Could you check a few things on this model? Use its own coordinates, in mm. Face numbers are marked on the shaded views. Round coordinates to 2 decimals unless told otherwise and drop trailing zeros. Loops run counter-clockwise (first coordinate to the right, second up) from the corner with the lowest first, then second, coordinate; pieces in that order, holes last. Notation, with made-up numbers: M 73.25,64.5 L 84.25,64.5 A23 ccw 84.25,88.5 Z; hole C -8.5,51 d5. An arc over 180 degrees is marked long. Answer in a Markdown table with one row per item.
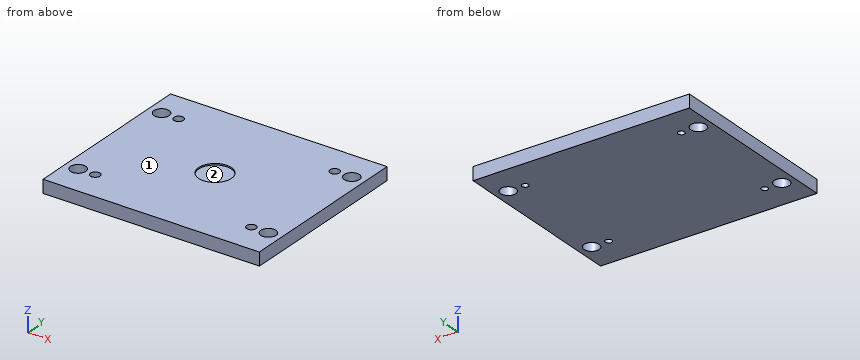
```python
from build123d import *

# Parameters (mm, degrees)
SZKIC1_W                    = 596
SZKIC1_H                    = 496
DODANIE_WYCI_GNI_CIE1_DEPTH = 36
SZKIC2_R                    = 45
WYTNIJ_WYCI_GNI_CIE1_DEPTH  = 4
SZKIC3_R                    = 21
WYTNIJ_WYCI_GNI_CIE2_DEPTH  = 36
SZKIC4_R                    = 21
WYTNIJ_WYCI_GNI_CIE3_DEPTH  = 36
SZKIC5_R                    = 21
WYTNIJ_WYCI_GNI_CIE4_DEPTH  = 36
SZKIC6_R                    = 21
WYTNIJ_WYCI_GNI_CIE5_DEPTH  = 36
SZKIC7_W                    = 15
SZKIC7_H                    = 9
SZKIC8_W                    = 15
SZKIC8_H                    = 9
SZKIC9_W                    = 15
SZKIC9_H                    = 9
SZKIC10_W                   = 15
SZKIC10_H                   = 9
SZKIC11_W                   = 21
SZKIC11_H                   = 13
SZKIC12_W                   = 21
SZKIC12_H                   = 13
SZKIC13_W                   = 21
SZKIC13_H                   = 13
SZKIC14_W                   = 21
SZKIC14_H                   = 13


with BuildPart() as part:
    # Szkic1 → Dodanie-wyci_gni_cie1 (new body)
    with BuildSketch(Plane.XY):
        Rectangle(SZKIC1_W, SZKIC1_H)
    extrude(amount=DODANIE_WYCI_GNI_CIE1_DEPTH)

    # Szkic2 → Wytnij-wyci_gni_cie1 (cut)
    with BuildSketch(Plane.XY.offset(36)):
        Circle(SZKIC2_R)
    extrude(amount=-WYTNIJ_WYCI_GNI_CIE1_DEPTH, mode=Mode.SUBTRACT)

    # Szkic3 → Wytnij-wyci_gni_cie2 (cut)
    with BuildSketch(Plane.XY.offset(36)):
        with Locations((262, 162)):
            Circle(SZKIC3_R)
    extrude(amount=-WYTNIJ_WYCI_GNI_CIE2_DEPTH, mode=Mode.SUBTRACT)

    # Szkic4 → Wytnij-wyci_gni_cie3 (cut)
    with BuildSketch(Plane.XY.offset(36)):
        with Locations((262, -162)):
            Circle(SZKIC4_R)
    extrude(amount=-WYTNIJ_WYCI_GNI_CIE3_DEPTH, mode=Mode.SUBTRACT)

    # Szkic5 → Wytnij-wyci_gni_cie4 (cut)
    with BuildSketch(Plane.XY.offset(36)):
        with Locations((-262, -162)):
            Circle(SZKIC5_R)
    extrude(amount=-WYTNIJ_WYCI_GNI_CIE4_DEPTH, mode=Mode.SUBTRACT)

    # Szkic6 → Wytnij-wyci_gni_cie5 (cut)
    with BuildSketch(Plane.XY.offset(36)):
        with Locations((-262, 162)):
            Circle(SZKIC6_R)
    extrude(amount=-WYTNIJ_WYCI_GNI_CIE5_DEPTH, mode=Mode.SUBTRACT)

    # Szkic7 → Wyci_cie-obr_t1 (revolve, cut)
    with BuildSketch(Plane(origin=(215, 0, 0), x_dir=(0, 0, -1), z_dir=(1, 0, 0)), mode=Mode.PRIVATE) as wyci_cie_obr_t1_sk:
        with Locations((-7.5, 166.5)):
            Rectangle(SZKIC7_W, SZKIC7_H)
    revolve(wyci_cie_obr_t1_sk.sketch.rotate(Axis((215, 162, 0), (0, 0, 1)), 270), axis=Axis((215, 162, 0), (0, 0, 1)), mode=Mode.SUBTRACT)

    # Szkic8 → Wyci_cie-obr_t2 (revolve, cut)
    with BuildSketch(Plane(origin=(215, 0, 0), x_dir=(0, 0, -1), z_dir=(1, 0, 0)), mode=Mode.PRIVATE) as wyci_cie_obr_t2_sk:
        with Locations((-7.5, -166.5)):
            Rectangle(SZKIC8_W, SZKIC8_H)
    revolve(wyci_cie_obr_t2_sk.sketch.rotate(Axis((215, -162, 15), (0, 0, -1)), 90), axis=Axis((215, -162, 15), (0, 0, -1)), mode=Mode.SUBTRACT)

    # Szkic9 → Wyci_cie-obr_t3 (revolve, cut)
    with BuildSketch(Plane(origin=(-215, 0, 0), x_dir=(0, 0, -1), z_dir=(1, 0, 0)), mode=Mode.PRIVATE) as wyci_cie_obr_t3_sk:
        with Locations((-7.5, 166.5)):
            Rectangle(SZKIC9_W, SZKIC9_H)
    revolve(wyci_cie_obr_t3_sk.sketch.rotate(Axis((-215, 162, 0), (0, 0, 1)), 270), axis=Axis((-215, 162, 0), (0, 0, 1)), mode=Mode.SUBTRACT)

    # Szkic10 → Wyci_cie-obr_t4 (revolve, cut)
    with BuildSketch(Plane(origin=(-215, 0, 0), x_dir=(0, 0, -1), z_dir=(1, 0, 0)), mode=Mode.PRIVATE) as wyci_cie_obr_t4_sk:
        with Locations((-7.5, -166.5)):
            Rectangle(SZKIC10_W, SZKIC10_H)
    revolve(wyci_cie_obr_t4_sk.sketch.rotate(Axis((-215, -162, 15), (0, 0, -1)), 90), axis=Axis((-215, -162, 15), (0, 0, -1)), mode=Mode.SUBTRACT)

    # Szkic11 → Wyci_cie-obr_t5 (revolve, cut)
    with BuildSketch(Plane(origin=(215, 0, 0), x_dir=(0, 0, -1), z_dir=(1, 0, 0)), mode=Mode.PRIVATE) as wyci_cie_obr_t5_sk:
        with Locations((-25.5, 168.5)):
            Rectangle(SZKIC11_W, SZKIC11_H)
    revolve(wyci_cie_obr_t5_sk.sketch.rotate(Axis((215, 162, 15), (0, 0, 1)), 270), axis=Axis((215, 162, 15), (0, 0, 1)), mode=Mode.SUBTRACT)

    # Szkic12 → Wyci_cie-obr_t6 (revolve, cut)
    with BuildSketch(Plane(origin=(215, 0, 0), x_dir=(0, 0, -1), z_dir=(1, 0, 0)), mode=Mode.PRIVATE) as wyci_cie_obr_t6_sk:
        with Locations((-25.5, -168.5)):
            Rectangle(SZKIC12_W, SZKIC12_H)
    revolve(wyci_cie_obr_t6_sk.sketch.rotate(Axis((215, -162, 36), (0, 0, -1)), 90), axis=Axis((215, -162, 36), (0, 0, -1)), mode=Mode.SUBTRACT)

    # Szkic13 → Wyci_cie-obr_t7 (revolve, cut)
    with BuildSketch(Plane(origin=(-215, 0, 0), x_dir=(0, 0, -1), z_dir=(1, 0, 0)), mode=Mode.PRIVATE) as wyci_cie_obr_t7_sk:
        with Locations((-25.5, -168.5)):
            Rectangle(SZKIC13_W, SZKIC13_H)
    revolve(wyci_cie_obr_t7_sk.sketch.rotate(Axis((-215, -162, 36), (0, 0, -1)), 90), axis=Axis((-215, -162, 36), (0, 0, -1)), mode=Mode.SUBTRACT)

    # Szkic14 → Wyci_cie-obr_t8 (revolve, cut)
    with BuildSketch(Plane(origin=(-215, 0, 0), x_dir=(0, 0, -1), z_dir=(1, 0, 0)), mode=Mode.PRIVATE) as wyci_cie_obr_t8_sk:
        with Locations((-25.5, 168.5)):
            Rectangle(SZKIC14_W, SZKIC14_H)
    revolve(wyci_cie_obr_t8_sk.sketch.rotate(Axis((-215, 162, 15), (0, 0, 1)), 270), axis=Axis((-215, 162, 15), (0, 0, 1)), mode=Mode.SUBTRACT)


solid = part.part
```
1) I want a section at C-C, the plane z = 26.5. State how many separate pieces and enclosed holes the cut face has, plus the area to 3 significant figures.
Computed:
| item | result |
|---|---|
| separate pieces | 1 |
| enclosed holes | 8 |
| area | 288,000 mm² |
2) I want a section at B-B, the plane y = 0. Please give me the cut outline in (x, z), plus the area to 3 significant figures.
Computed:
| item | result |
|---|---|
| outline | M -298,0 L 298,0 L 298,36 L 45,36 L 45,32 L -45,32 L -45,36 L -298,36 Z |
| area | 21,100 mm² |
3) I want a section at D-D, the plane x = 0. Please give me the cut outline in (y, z).
Computed:
| item | result |
|---|---|
| outline | M -248,0 L 248,0 L 248,36 L 45,36 L 45,32 L -45,32 L -45,36 L -248,36 Z |
4) I need wall thicknesses on line 1 (Y direction, x = 215, z = 22.5); line 2 (Y direction, x = 262, z = 25.5); line 3 (X direction, y = 147.5, z = 12). Which ranges of each line are inside material? Lowest first, please.
Computed:
| item | result |
|---|---|
| line 1 | y = -248 to -175, -149 to 149, 175 to 248 |
| line 2 | y = -248 to -183, -141 to 141, 183 to 248 |
| line 3 | x = -298 to -277.19, -246.81 to 246.81, 277.19 to 298 |
5) Will these pins go through, and if not, where does the flat tip stop? P1, Ø8, axis at x = -212, y = 167, coming from the +Z side; P2, Ø16, axis at x = 215, y = 162, coming from the -Z side.
Computed:
| item | result |
|---|---|
| P1 | stops at z = 15 |
| P2 | passes through |
6) I want a section at A-A, the plane x = -262. Please give me the cut outline in (y, z).
Computed:
| item | result |
|---|---|
| outline | M -248,0 L -183,0 L -183,36 L -248,36 Z; M -141,0 L 141,0 L 141,36 L -141,36 Z; M 183,0 L 248,0 L 248,36 L 183,36 Z |
7) If we mould it in two halves opening along X, with no side actions, what happens to the marked faces 1 and 2? For each: released by +X, released by -X, zero draft, split by the parting line, or undercut.
Computed:
| item | result |
|---|---|
| face 1 | zero draft |
| face 2 | undercut |
